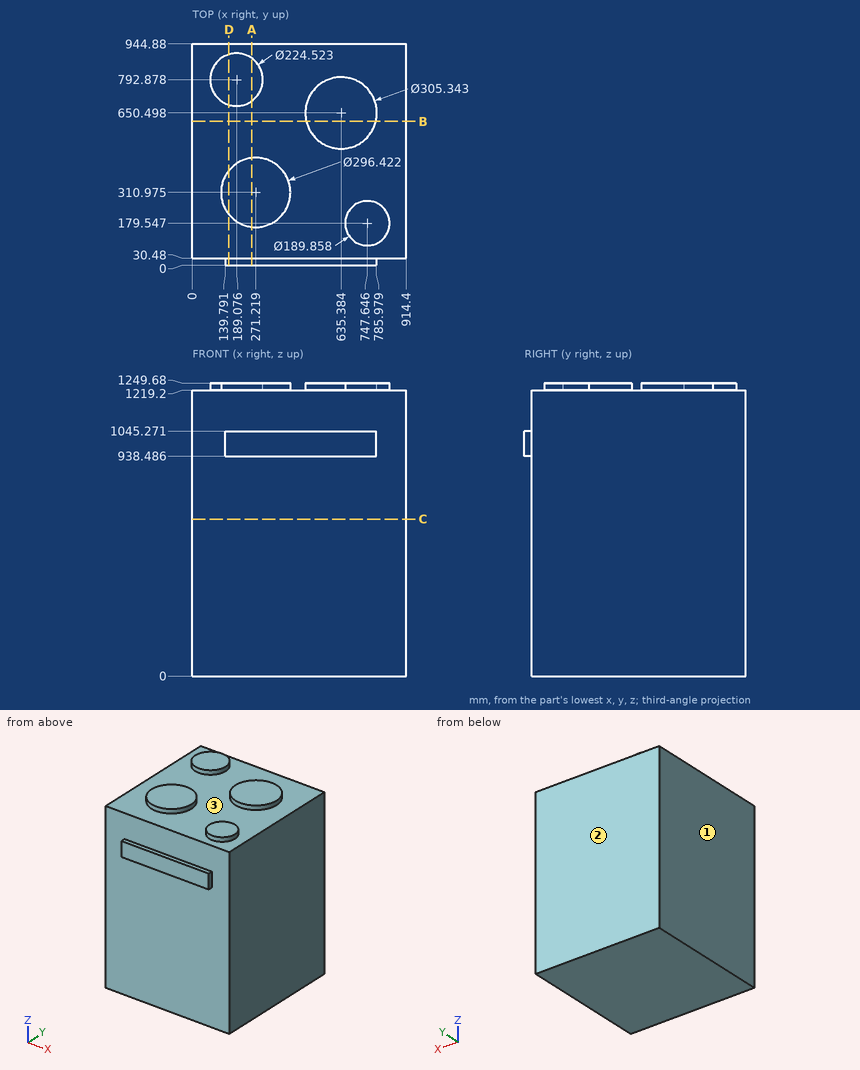
Verification items for this drawing (mm, ordinates from the low corner). Give positions to 0.01 mm unless a question says otherwise; leave off trailing zeros. Loops run counter-clockwise (first coordinate to the right, second up) from the corner with the lowest first, then second, coordinate; pieces in that order, holes last. Notation, with made-up numbers: M 79,0 L 101,0 A20 cw 101,32 Z; hole C 60,30 d11. An arc over 180 degrees is marked long. Answer as a JSON object with one key per item and string values. Group by question number.
Item 1: Gauge pin test, flat ends, axial feed: pin 1 (1 mm diameter, centred on x = 751, z = 1093.5, fed in from -Y); pin 2 (9 mm diameter, centred on x = 545, y = 17.5, fed in from +Z); pin 3 (24.5 mm diameter, centred on y = 12, z = 1007, fed in from -X). Record the tip position at first contact, or that the pin passes through.
Item 2: Sectioned sample at B-B on y = 614.5. Record the boundary of the cut face in (x, z).
Item 3: Sectioned sample at A-A on x = 254.5. Record the boundary of the cut face in (y, z) (1 decimal), plus the area to 3 significant figures.
Item 4: Mould release check, pull along Y, two halves, no side actions. Record for the marked faces 1, 2 and 3: pulls with the +Y half, pulls with the -Y half, needs draft (parallel to the pull), parting line crosses it, or undercut.
Item 5: Sectioned sample at C-C on z = 670. Record the boundary of the cut face in (x, y).
Item 6: Material ranges on L1, parallel to Y at x = 114.5, z = 152; L2, parallel to Z at x = 684.5, y = 441, recorded low to high.
Item 7: Sectioned sample at D-D on x = 156.5. Record the boundary of the cut face in (y, z) (1 decimal).
Findings below:
{
 "1": {"pin 1": "y = 30.48", "pin 2": "z = 1045.27", "pin 3": "x = 139.79"},
 "2": {"outline": "M 0,0 L 914.4,0 L 914.4,1219.2 L 783.75,1219.2 L 783.75,1249.68 L 487.02,1249.68 L 487.02,1219.2 L 0,1219.2 Z"},
 "3": {"outline": "M 0,938.5 L 30.5,938.5 L 30.5,0 L 944.9,0 L 944.9,1219.2 L 884.1,1219.2 L 884.1,1249.7 L 701.7,1249.7 L 701.7,1219.2 L 458.2,1219.2 L 458.2,1249.7 L 163.7,1249.7 L 163.7,1219.2 L 30.5,1219.2 L 30.5,1045.3 L 0,1045.3 Z", "area": "1,130,000 mm2"},
 "4": {"face 1": "needs draft", "face 2": "pulls with the +Y half", "face 3": "undercut"},
 "5": {"outline": "M 0,30.48 L 914.4,30.48 L 914.4,944.88 L 0,944.88 Z"},
 "6": {"L1": "30.48 to 944.88", "L2": "0 to 1219.2"},
 "7": {"outline": "M 0,938.5 L 30.5,938.5 L 30.5,0 L 944.9,0 L 944.9,1219.2 L 900.3,1219.2 L 900.3,1249.7 L 685.4,1249.7 L 685.4,1219.2 L 404.8,1219.2 L 404.8,1249.7 L 217.1,1249.7 L 217.1,1219.2 L 30.5,1219.2 L 30.5,1045.3 L 0,1045.3 Z"}
}
